For this review, use the dimensioned drawing (mm, ordinates from the lowest corner) and the shaded views. A direction names the side the tool comes from. Give positions to 0.01 mm unless a question says otherwise; leave off trailing zeros. Write each loop counter-clockwise with the first axis right and the second up, starting at its lowest first coordinate (ties: lowest second). Pieces come first, ordered by that corner, then holes. Notation, with made-up numbers: (4, -35.75) - (48, -35.75) arc R20 ccw to (48, 2.25) - close; hole circle Ø7 at (-29, 55.5). An arc over 180 degrees is marked (long way). Use a Markdown table: item, result. Add a question column.
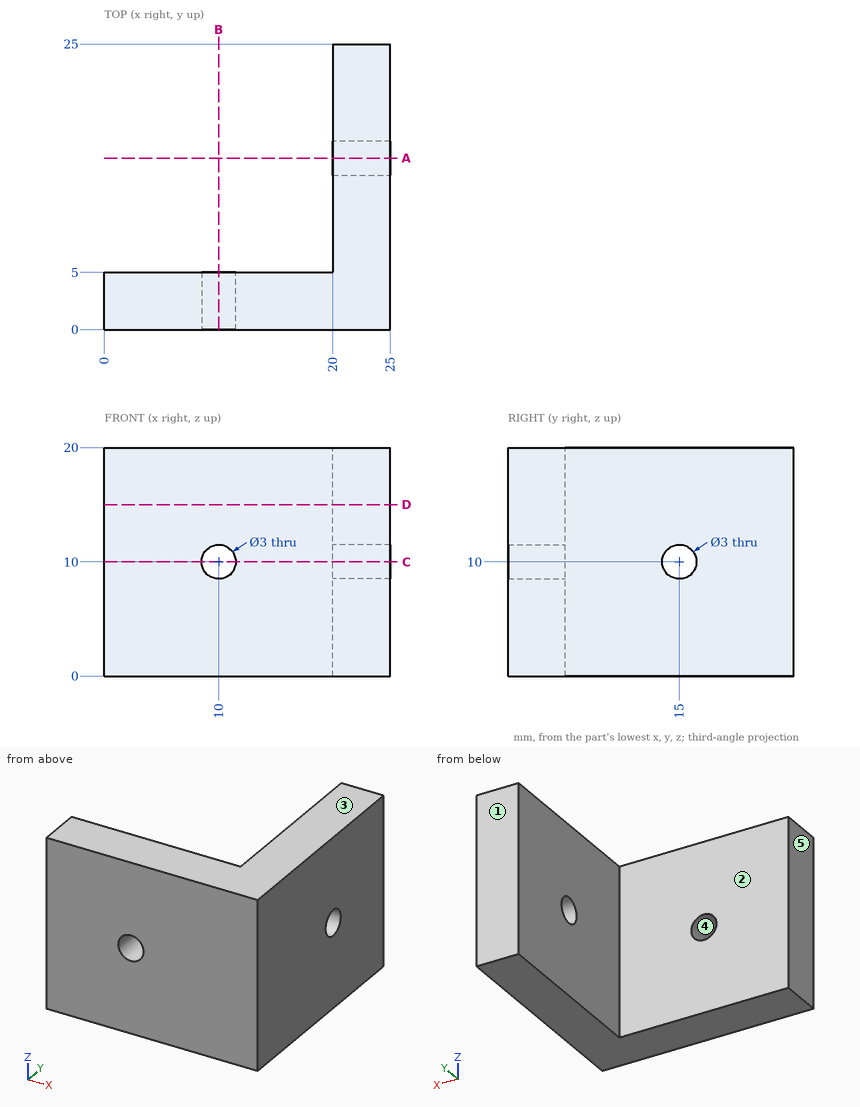
(1) Tool access review of the marked faces 1 and 2: name each direction out of +Z, -Z, +X, -X, +Y, -Y from which nothing blocks a thin tool from reaching the whole face with its end or side.
(2) For line 1 along Z through (x, y) = (10, 1.6); line 2 along X through (y, z) = (17, 6.25); line 3 along Y through (x, z) = (9, 18), list the stretches that pass through material, from the lowest coordinate up.
(3) Add section A-A (y = 15). State the section outline as (x, z) points, and give its area (3 significant figures).
(4) Insertion check: pin 1 (1 mm diameter, centred on x = 12, z = 13.5, fed in from +Y); pin 2 (1 mm diameter, centred on y = 13.5, z = 2.5, fed in from -X); pin 3 (1.8 mm diameter, centred on y = 15, z = 10, fed in from -X). Each pin has a flat end and moves straight along its axis. Give the tip position at first contact, or say it passes through.
(5) Mouldability with a two-part tool opening along Z and no side actions: class the marked faces 3, 4 and 5 as +Z half, -Z half, draft (parallel to the pull), parting line (faces both ways), or undercut.
(6) Add section B-B (x = 10). State the section outline as (y, z) points, and give its area (3 significant figures).
(7) Add section C-C (z = 10). State the section outline as (x, y) points, and give its area (3 significant figures).
(8) Add section D-D (z = 15). State the section outline as (x, y) points, and give its area (3 significant figures).
Answers follow:
| question | item | result |
|---|---|---|
| 1 | face 1 | +Z, -Z, +X, -X, +Y |
| 1 | face 2 | +Z, -Z, -X, +Y |
| 2 | line 1 | 0 to 8.5, 11.5 to 20 |
| 2 | line 2 | 20 to 25 |
| 2 | line 3 | 0 to 5 |
| 3 | outline | (20, 0) - (25, 0) - (25, 8.5) - (20, 8.5) - close; (20, 11.5) - (25, 11.5) - (25, 20) - (20, 20) - close |
| 3 | area | 85.0 mm^2 |
| 4 | pin 1 | y = 5 |
| 4 | pin 2 | x = 20 |
| 4 | pin 3 | through |
| 5 | face 3 | +Z half |
| 5 | face 4 | undercut |
| 5 | face 5 | draft |
| 6 | outline | (0, 0) - (5, 0) - (5, 8.5) - (0, 8.5) - close; (0, 11.5) - (5, 11.5) - (5, 20) - (0, 20) - close |
| 6 | area | 85.0 mm^2 |
| 7 | outline | (0, 0) - (8.5, 0) - (8.5, 5) - (0, 5) - close; (11.5, 0) - (25, 0) - (25, 13.5) - (20, 13.5) - (20, 5) - (11.5, 5) - close; (20, 16.5) - (25, 16.5) - (25, 25) - (20, 25) - close |
| 7 | area | 195 mm^2 |
| 8 | outline | (0, 0) - (25, 0) - (25, 25) - (20, 25) - (20, 5) - (0, 5) - close |
| 8 | area | 225 mm^2 |
